from build123d import *

# Parameters (mm, degrees)
SKETCH1_R           = 1.675
BOSS_EXTRUDE1_DEPTH = 6
SKETCH2_R           = 3.5
CUT_EXTRUDE1_DEPTH  = 3
FILLET1_R           = 0.75


with BuildPart() as part:
    # Sketch1 → Boss-Extrude1 (new body)
    with BuildSketch(Plane.XY):
        with BuildLine():
            Line((-10.468847051, 3), (10.468847051, 3))
            ThreePointArc((10.468847051, 3), (11.081219486, 3.130693606), (11.586881039, 3.5))
            ThreePointArc((11.586881039, 3.5), (20.75, 0), (11.586881039, -3.5))
            ThreePointArc((11.586881039, -3.5), (11.081219486, -3.130693606), (10.468847051, -3))
            Line((10.468847051, -3), (-10.468847051, -3))
            ThreePointArc((-10.468847051, -3), (-11.081219486, -3.130693606), (-11.586881039, -3.5))
            ThreePointArc((-11.586881039, -3.5), (-20.75, 0), (-11.586881039, 3.5))
            ThreePointArc((-11.586881039, 3.5), (-11.081219486, 3.130693606), (-10.468847051, 3))
        make_face()
        with Locations((15.5, 0)):
            Circle(SKETCH1_R, mode=Mode.SUBTRACT)
        with Locations((-15.5, 0)):
            Circle(SKETCH1_R, mode=Mode.SUBTRACT)
    extrude(amount=BOSS_EXTRUDE1_DEPTH)

    # Sketch2 → Cut-Extrude1 (cut)
    with BuildSketch(Plane.XY.offset(6)):
        with Locations((-15.5, 0)):
            Circle(SKETCH2_R)
        with Locations((15.5, 0)):
            Circle(SKETCH2_R)
    extrude(amount=-CUT_EXTRUDE1_DEPTH, mode=Mode.SUBTRACT)

    # Fillet1
    fillet1_edges = [part.edges().sort_by_distance(p)[0] for p in [
        (11.081219486, 3.130693606, 6),
        (0, 3, 6),
        (-11.081219486, 3.130693606, 6),
        (-20.75, 0, 6),
        (-11.081219486, -3.130693606, 6),
        (0, -3, 6),
        (-19, 0, 6),
        (12, 0, 6),
        (11.081219486, -3.130693606, 6),
        (20.75, 0, 6),
    ]]
    fillet(fillet1_edges, radius=FILLET1_R)


solid = part.part
Design review of the part built by this model. Coordinates are the model's own, in mm. A direction names the side the tool comes from. Round coordinates to 2 decimals unless told otherwise and drop trailing zeros. Order: outer loops, then holes, each group sorted by start corner. A loop starts at its lowest first (then second) coordinate and runs counter-clockwise, first axis right, second up. Notation, with made-up numbers: M 11.5,-9.5 L 46.5,-9.5 A34 ccw 46.5,20.5 Z; hole C 5,10 d2. An arc over 180 degrees is marked long. Answer as CSV lines item,"result". Start each with the question number.
1) Add section B-B (y = 0). Give the boundary of the cut face in (x, z) (3 decimals), then the cut area to 3 significant figures.
2) The part is to be moulded in two halves that separate along X. For faces 4 (the face through (0, 0, 6)), 5 (the face through (20.747, 0.177, 2.588)), say which applies: +X half, -X half, draft (parallel to the pull), parting line (faces both ways), or undercut.
3) Add section D-D (z = 1.35). Give the boundary of the cut face in (x, y) (3 decimals).
4) Wall thickness on line 1 along X through (y, z) = (0, 2.2) (3 decimals); line 2 along Y through (x, z) = (15.5, 4.2); line 3 along X through (y, z) = (2.75, 5.7): over which ranges is each line inside the solid? List them lowest first. Write a range as [from, to].
5) Tool access review of faces 1 (the face through (-11.073, -3.127, 2.588)), 2 (the face through (-11.089, 3.134, 2.588)), 3 (the face through (18.84, 1.05, 4.14)): name each direction out of +Z, -Z, +X, -X, +Y, -Y from which nothing blocks a thin tool from reaching the whole face with its end or side.
6) Add section C-C (x = -6). Give the boundary of the cut face in (y, z).
7) Add section A-A (z = 3.65). Give the boundary of the cut face in (x, y), then the cut area to 3 significant figures.
8) For pin 1 Ø1 at (x, z) = (7, 2.5) entering from -Y; pin 2 Ø5.5 at (x, y) = (-17, 0.5) entering from +Z; pin 3 Ø2.5 at (x, y) = (-15.5, 0) entering from +Z; pin 4 Ø3 at (y, z) = (2, 5) entering from -X, all flat-tipped, find the tip position at first contact; note any pin that passes through.
Resolved:
1,outline,"M -20.75,0 L -17.175,0 L -17.175,3 L -19,3 L -19,5.25 A0.75 ccw -19.75,6 L -20,6 A0.75 ccw -20.75,5.25 Z; M -13.825,0 L 13.825,0 L 13.825,3 L 12,3 L 12,5.25 A0.75 ccw 11.25,6 L -11.25,6 A0.75 ccw -12,5.25 L -12,3 L -13.825,3 Z; M 17.175,0 L 20.75,0 L 20.75,5.25 A0.75 ccw 20,6 L 19.75,6 A0.75 ccw 19,5.25 L 19,3 L 17.175,3 Z"
1,area,"186 mm^2"
2,face 4,"draft"
2,face 5,"undercut"
3,outline,"M -11.587,-3.5 A1.5 cw -10.469,-3 L 10.469,-3 A1.5 cw 11.587,-3.5 A5.25 ccw long 11.587,3.5 A1.5 cw 10.469,3 L -10.469,3 A1.5 cw -11.587,3.5 A5.25 ccw long Z; hole C -15.5,0 d3.35; hole C 15.5,0 d3.35"
4,line 1,"[-20.75, -17.175], [-13.825, 13.825], [17.175, 20.75]"
4,line 2,"[-5.25, -3.5], [3.5, 5.25]"
4,line 3,"[-19.8, -17.9], [-13.1, 13.1], [17.9, 19.8]"
5,face 1,"+Z, -Z, -Y"
5,face 2,"+Z, -Z, +Y"
5,face 3,"+Z"
6,outline,"M -3,0 L 3,0 L 3,5.25 A0.75 ccw 2.25,6 L -2.25,6 A0.75 ccw -3,5.25 Z"
7,outline,"M -11.59,-3.5 A1.5 cw -10.47,-3 L 10.47,-3 A1.5 cw 11.59,-3.5 A5.25 ccw long 11.59,3.5 A1.5 cw 10.47,3 L -10.47,3 A1.5 cw -11.59,3.5 A5.25 ccw long Z; hole C -15.5,0 d7; hole C 15.5,0 d7"
7,area,"223 mm^2"
8,pin 1,"y = -3"
8,pin 2,"z = 6"
8,pin 3,"through"
8,pin 4,"x = -20.73"
